from build123d import *

# Parameters (mm, degrees)
SKETCH1_W           = 106
SKETCH1_H           = 110
SKETCH1_R           = 1.1
BOSS_EXTRUDE1_DEPTH = 1
BOSS_EXTRUDE3_DEPTH = 5
SKETCH3_W           = 10.16
SKETCH3_H           = 13
BOSS_EXTRUDE4_DEPTH = 5
SKETCH4_W           = 13.5
SKETCH4_H           = 9.2
BOSS_EXTRUDE5_DEPTH = 6


with BuildPart() as part:
    # Sketch1 → Boss-Extrude1 (new body)
    with BuildSketch(Plane(origin=(0, 0, 0), x_dir=(1, 0, 0), z_dir=(0, 1, 0))):
        with Locations((8.955727632, 44.943820005)):
            Rectangle(SKETCH1_W, SKETCH1_H)
        with Locations(Location((-40.544272368, -6.556179995, 0), (0, 0, 270))):
            Circle(SKETCH1_R, mode=Mode.SUBTRACT)
        with Locations(Location((58.455727632, -6.556179995, 0), (0, 0, 270))):
            Circle(SKETCH1_R, mode=Mode.SUBTRACT)
        with Locations(Location((-40.544272368, 96.443820005, 0), (0, 0, 270))):
            Circle(SKETCH1_R, mode=Mode.SUBTRACT)
        with Locations(Location((58.455727632, 96.443820005, 0), (0, 0, 270))):
            Circle(SKETCH1_R, mode=Mode.SUBTRACT)
    extrude(amount=BOSS_EXTRUDE1_DEPTH)

    # 3DSketch1 → Boss-Extrude3 (add)
    with BuildSketch(Plane(origin=(-17.624272368, 1, -0.613820005), x_dir=(0.47206668121683765, 0, 0.8815628443196325), z_dir=(0, -1, 0))):
        Polygon((0, 0), (3.597148111, -6.717508874), (16.141787386, 0), (12.544639275, 6.717508874), align=None)
    extrude(amount=-BOSS_EXTRUDE3_DEPTH)

    # Sketch3 → Boss-Extrude4 (add)
    with BuildSketch(Plane(origin=(0, 1, 0), x_dir=(1, 0, 0), z_dir=(0, 1, 0))):
        with Locations((6.825727632, -4.886179995)):
            Rectangle(SKETCH3_W, SKETCH3_H)
    extrude(amount=BOSS_EXTRUDE4_DEPTH)

    # Sketch4 → Boss-Extrude5 (add)
    with BuildSketch(Plane(origin=(0, 1, 0), x_dir=(-1, 0, 0), z_dir=(0, 1, 0))):
        with Locations((-41.985727632, 10.746179995)):
            Rectangle(SKETCH4_W, SKETCH4_H)
        with Locations((-25.225727632, 10.746179995)):
            Rectangle(SKETCH4_W, SKETCH4_H)
    extrude(amount=BOSS_EXTRUDE5_DEPTH)


solid = part.part
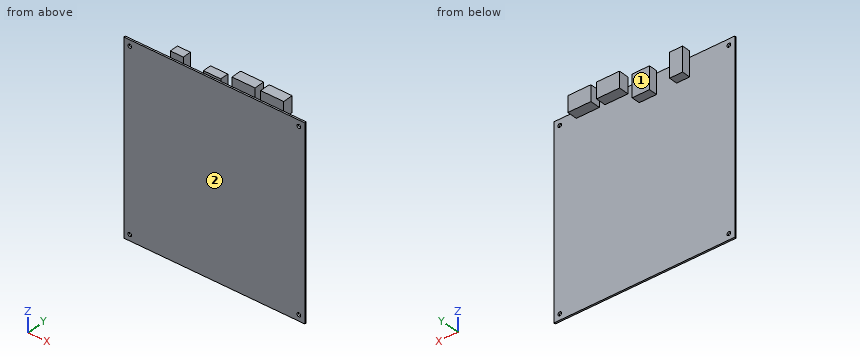
CAD build for the part. Positions are in the model's coordinates, mm. Face numbers are marked on the shaded views. A direction names the side the tool comes from. Coordinates: 2 decimals unless noted, no trailing zeros. Write each loop counter-clockwise with the first axis right and the second up, starting at its lowest first coordinate (ties: lowest second). Pieces come first, ordered by that corner, then holes. Notation, with made-up numbers: M 25.5,15.25 L 78.5,15.25 A20 cw 78.5,22.25 Z; hole C -5,73 d3. An arc over 180 degrees is marked long. Answer as a JSON object with one key per item and string values. Group by question number.
1) Saw through at D-D (x = -12.5). Write the cut outline in (y, z), plus the area to 3 significant figures.
2) Wall check: line 1 (X direction, y = 4.75, z = 9); line 2 (Y direction, x = -25.5, z = -26); line 3 (Z direction, x = 25, y = 4.75). Give the ranges that are in metal, low to high. Write a range as from..to.
3) Saw through at C-C (z = 2). Write the cut outline in (x, y).
4) Saw through at A-A (y = 3). Write the cut outline in (x, z), plus the area to 3 significant figures.
5) Pin check, flat tips, straight feed: pin 1 Ø3 at (x, y) = (41, 3.5) entering from -Z; pin 2 Ø1.5 at (x, y) = (-15.5, 2.5) entering from -Z; pin 3 Ø8 at (x, z) = (-18, -72.5) entering from +Y. Stop position of each tip, or through.
6) Saw through at B-B (x = 24.5). Write the cut outline in (y, z).
7) Tool access for the marked faces 1 and 2: list every direction of +Z, -Z, +X, -X, +Y, -Y with a clear straight run to the whole face (end or side of a thin tool).
Values follow:
{
 "1": {"outline": "M 0,-99.94 L 1,-99.94 L 1,-0.61 L 6,-0.61 L 6,13.62 L 1,13.62 L 1,10.06 L 0,10.06 Z", "area": "181 mm2"},
 "2": {"line 1": "x = -17.62..-10, 1.75..11.91, 18.48..31.98, 35.24..48.74", "line 2": "y = 0..1", "line 3": "z = 6.15..15.35"},
 "3": {"outline": "M -44.04,0 L 61.96,0 L 61.96,1 L 11.91,1 L 11.91,6 L 1.75,6 L 1.75,1 L -10,1 L -10,6 L -17.62,6 L -17.62,1 L -44.04,1 Z"},
 "4": {"outline": "M -17.62,-0.61 L -10,-0.61 L -10,13.62 L -17.62,13.62 Z; M 1.75,-1.61 L 11.91,-1.61 L 11.91,11.39 L 1.75,11.39 Z; M 18.48,6.15 L 31.98,6.15 L 31.98,15.35 L 18.48,15.35 Z; M 35.24,6.15 L 48.74,6.15 L 48.74,15.35 L 35.24,15.35 Z", "area": "489 mm2"},
 "5": {"pin 1": "stops at z = 6.15", "pin 2": "stops at z = -0.61", "pin 3": "stops at y = 1"},
 "6": {"outline": "M 0,-99.94 L 1,-99.94 L 1,6.15 L 7,6.15 L 7,15.35 L 1,15.35 L 1,10.06 L 0,10.06 Z"},
 "7": {"face 1": "+Z, -Z, -X, +Y", "face 2": "+Z, -Z, +X, -X, -Y"}
}
